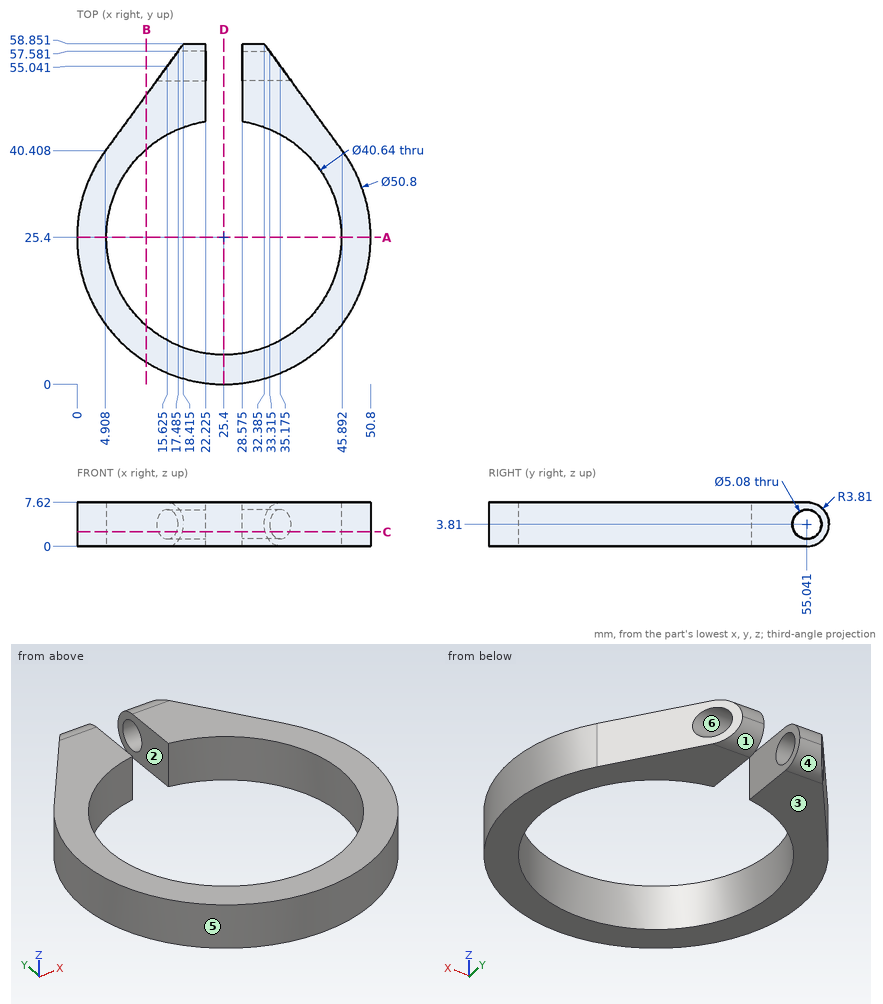
Here's the drawing with two shaded views (mm, measured from the low corner). I have some questions. A direction names the side the tool comes from. Round coordinates to 2 decimals unless told otherwise and drop trailing zeros. Write each loop counter-clockwise with the first axis right and the second up, starting at its lowest first coordinate (ties: lowest second). Pieces come first, ordered by that corner, then holes. Notation, with made-up numbers: M 71,84.25 L 116,84.25 A18 ccw 116,117.25 Z; hole C 44,26 d11. An arc over 180 degrees is marked long. Write each question's results on one line, items separated by ' | '. Start each with the question number.
1. Imagine slicing it at A-A on y = 25.4. List the corners of the cut face in (x, z) for me.
2. Imagine slicing it at B-B on x = 12. List the corners of the cut face in (y, z) for me (1 decimal).
3. Imagine slicing it at C-C on z = 2.5. List the corners of the cut face in (x, y) for me (1 decimal), and give its area (3 significant figures).
4. Imagine slicing it at D-D on x = 25.4. List the corners of the cut face in (y, z) for me, and give its area (3 significant figures).
5. I need wall thicknesses on L1, parallel to Y at x = 17, z = 5; L2, parallel to X at y = 52, z = 3 (1 decimal); L3, parallel to Y at x = 21.5, z = 4.5 (1 decimal). Which ranges of each line are inside material? Lowest first, please. Write a range as from..to.
6. On a 3-axis mill with a long thin cutter (end or side, diameter ignored), from which of +Z, -Z, +X, -X, +Y, -Y can I reach the whole of each face in a straight line? I mean the marked faces 1 and 2. Say none if no direction works.
7. I'm going to push flat-ended pins straight in: pin 1 Ø2.5 at (y, z) = (50, 5) entering from +X; pin 2 Ø5 at (x, y) = (9, 50) entering from +Z; pin 3 Ø2.5 at (y, z) = (49.5, 4.5) entering from -X; pin 4 Ø1.5 at (y, z) = (29, 1) entering from -X. Where does each tip first touch, or does it pass through?
8. Thinking about a two-plate mould opening in Y: for the marked faces 3, 4, 5 and 6, which applies, +Y half, -Y half, draft (parallel to the pull), parting line (faces both ways), or undercut?
Result sheet:
1) outline: M 0,0 L 5.08,0 L 5.08,7.62 L 0,7.62 Z; M 45.72,0 L 50.8,0 L 50.8,7.62 L 45.72,7.62 Z
2) outline: M 3.8,0 L 10.1,0 L 10.1,7.6 L 3.8,7.6 Z; M 40.7,0 L 50.1,0 L 50.1,7.6 L 40.7,7.6 Z
3) outline: M 4.9,40.4 A25.4 ccw long 45.9,40.4 L 36.8,52.9 L 28.6,52.9 L 28.6,45.5 A20.3 cw long 22.2,45.5 L 22.2,52.9 L 14,52.9 Z; M 17.2,57.2 L 22.2,57.2 L 22.2,58.6 L 18.2,58.6 Z; M 28.6,57.2 L 33.6,57.2 L 32.6,58.6 L 28.6,58.6 Z | area: 795 mm^2
4) outline: M 0,0 L 5.08,0 L 5.08,7.62 L 0,7.62 Z | area: 38.7 mm^2
5) L1: y = 1.43..6.9, 43.9..52.8 | L2: x = 13.4..22.2, 28.6..37.4 | L3: y = 0.3..5.5, 45.3..52.6, 57.5..58.8
6) face 1: -Z, +X, -X, +Y | face 2: +Z, -Z, +Y
7) pin 1: stops at x = 39.78 | pin 2: stops at z = 7.62 | pin 3: stops at x = 10.65 | pin 4: stops at x = 0.16
8) face 3: draft | face 4: +Y half | face 5: parting line | face 6: undercut
